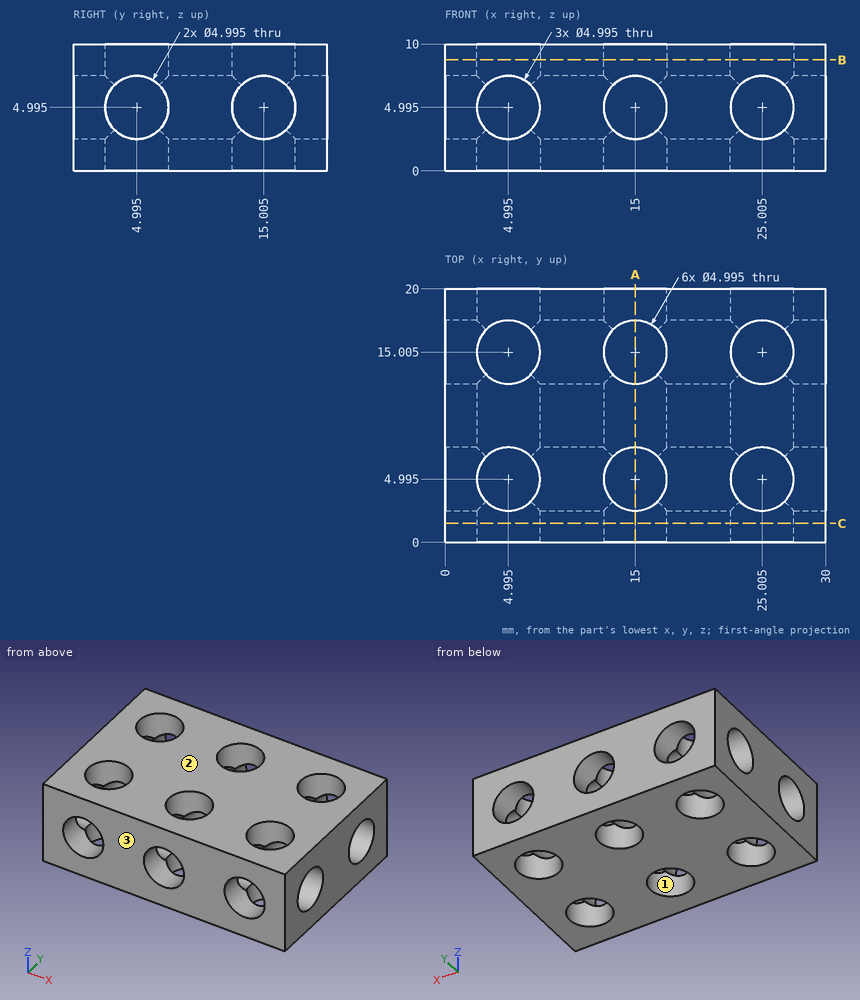
Verification items for this drawing (mm, ordinates from the low corner). Round coordinates to 2 decimals unless told otherwise and drop trailing zeros. Loops run counter-clockwise (first coordinate to the right, second up) from the corner with the lowest first, then second, coordinate; pieces in that order, holes last. Notation, with made-up numbers: (25.5, 69.5) -> (59.5, 69.5) arc R16 ccw to (59.5, 92.5) -> close; hole circle Ø7 at (-2, 15.5). An arc over 180 degrees is marked (long way). Write item = value, one per line. Start each with the question number.
1) Sectioned sample at C-C, the plane y = 1.5. Record the cut outline in (x, z) (1 decimal).
2) Release check for a two-part mould opening along Y. For the marked faces 1, 2 and 3 record: released by +Y, released by -Y, zero draft, split by the parting line, or undercut.
3) Sectioned sample at B-B, the plane z = 8.75. Record the cut outline in (x, y) (1 decimal), plus the area to 3 significant figures.
4) Sectioned sample at A-A, the plane x = 15. Record the cut outline in (y, z).
5) Thickness scan on probe 1 along Y at (x, z) = (15, 8); probe 2 along Y at (x, z) = (3, 7.5); probe 3 along X at (y, z) = (17, 7.5). Record the ranges inside material, lowest first.
Results are:
q1.outline = (0, 0) -> (30, 0) -> (30, 10) -> (0, 10) -> close; hole circle Ø5 at (5, 5); hole circle Ø5 at (15, 5); hole circle Ø5 at (25, 5)
q2.face_1 = undercut
q2.face_2 = zero draft
q2.face_3 = released by -Y
q3.outline = (0, 0) -> (30, 0) -> (30, 20) -> (0, 20) -> close; hole circle Ø5 at (5, 5); hole circle Ø5 at (5, 15); hole circle Ø5 at (15, 5); hole circle Ø5 at (15, 15); hole circle Ø5 at (25, 5); hole circle Ø5 at (25, 15)
q3.area = 482 mm^2
q4.outline = (0, 0) -> (2.5, 0) -> (2.5, 2.5) -> (0, 2.5) -> close; (0, 7.49) -> (2.5, 7.49) -> (2.5, 10) -> (0, 10) -> close; (7.49, 0) -> (12.51, 0) -> (12.51, 2.5) -> (7.49, 2.5) -> close; (7.49, 7.49) -> (12.51, 7.49) -> (12.51, 10) -> (7.49, 10) -> close; (17.5, 0) -> (20, 0) -> (20, 2.5) -> (17.5, 2.5) -> close; (17.5, 7.49) -> (20, 7.49) -> (20, 10) -> (17.5, 10) -> close
q5.probe_1 = 0 to 2.5, 7.49 to 12.51, 17.5 to 20
q5.probe_2 = 0 to 3.49, 6.5 to 13.5, 16.51 to 20
q5.probe_3 = 0 to 3.49, 6.5 to 13.5, 16.5 to 23.5, 26.51 to 30
